Could you check a few things on this model? Use its own coordinates, in mm. A direction names the side the tool comes from. Coordinates: 2 decimals unless noted, no trailing zeros. Order: outer loops, then holes, each group sorted by start corner. A loop starts at its lowest first (then second) coordinate and runs counter-clockwise, first axis right, second up. Notation, with made-up numbers: (34, 22.25) -> (63, 22.25) arc R14 cw to (63, 47.25) -> close; hole circle Ø1 at (-22, 2.25). An arc over 180 degrees is marked (long way). Return JSON: item names as keys, results as strings. Group by question number.
from build123d import *

# Parameters (mm, degrees)
F0_W     = 100
F0_H     = 70
F1_DEPTH = 30
F2_W     = 70
F2_H     = 60
F3_DEPTH = 13.9
F4_W     = 51.206012
F4_H     = 33.682036
F5_DEPTH = 3.8


with BuildPart() as f1:
    # F0 (on Front) → F1 (new body)
    with BuildSketch(Plane.XZ):
        Rectangle(F0_W, F0_H)
    extrude(amount=F1_DEPTH)

    # F2 (on face) → F3 (cut)
    with BuildSketch(Plane.XZ.offset(30)):
        Rectangle(F2_W, F2_H)
    extrude(amount=-F3_DEPTH, mode=Mode.SUBTRACT)

    # F4 (on face) → F5 (cut)
    with BuildSketch(Plane.XZ.offset(16.1)):
        Rectangle(F4_W, F4_H)
    extrude(amount=-F5_DEPTH, mode=Mode.SUBTRACT)


solid = f1.part
Q1. I want a section at B-B on y = -21. Please give me the cut outline in (x, z).
Q2. I want a section at D-D on z = 14.5. Please give me the cut outline in (x, y).
Q3. On a 3-axis mill with a long thin cutter (end or side, diameter ignored), from which of +Z, -Z, +X, -X, +Y, -Y can I reach the whole of each face in a straight line? I mean faces 4 (the flat face through (-1, -30, -31)), 5 (the flat face through (0, -16.1, 20)). Say none if no direction works.
Q4. I want a section at A-A on z = -18. Please give me the cut outline in (x, y).
Q5. I'm going to push flat-ended pins straight in: pin 1 Ø2 at (x, z) = (-12, 20) entering from -Y; pin 2 Ø12 at (x, z) = (-7, 1.5) entering from -Y. Where does each tip first touch, or does it pass through?
Q6. I want a section at C-C on x = 20.5. Please give me the cut outline in (y, z), and give its area (3 significant figures).
Q7. I need wall thicknesses on line 1 along X through (y, z) = (-19.5, -4.5); line 2 along Z through (x, y) = (-21, -12.5); line 3 along Z through (x, y) = (5, -21.75). Which ranges of each line are inside material? Lowest first, please. Write a range as from..to.
Q8. We'd pull the mould along X, two halves only. Please class faces 1 (the flat face through (0, -14, -16.841)), 2 (the flat face through (50, -15, 0)), 3 (the flat face through (-1, 0, 0)): pulls with the +X half, pulls with the -X half, needs draft (parallel to the pull), parting line crosses it, or undercut.
Response values:
{
 "1": {"outline": "(-50, -35) -> (50, -35) -> (50, 35) -> (-50, 35) -> close; hole (-35, -30) -> (35, -30) -> (35, 30) -> (-35, 30) -> close"},
 "2": {"outline": "(-50, -30) -> (-35, -30) -> (-35, -16.1) -> (-25.6, -16.1) -> (-25.6, -12.3) -> (25.6, -12.3) -> (25.6, -16.1) -> (35, -16.1) -> (35, -30) -> (50, -30) -> (50, 0) -> (-50, 0) -> close"},
 "3": {"face 4": "+Z, -Z, +X, -X, -Y", "face 5": "-Y"},
 "4": {"outline": "(-50, -30) -> (-35, -30) -> (-35, -16.1) -> (35, -16.1) -> (35, -30) -> (50, -30) -> (50, 0) -> (-50, 0) -> close"},
 "5": {"pin 1": "stops at y = -16.1", "pin 2": "stops at y = -12.3"},
 "6": {"outline": "(-30, -35) -> (0, -35) -> (0, 35) -> (-30, 35) -> (-30, 30) -> (-16.1, 30) -> (-16.1, 16.84) -> (-12.3, 16.84) -> (-12.3, -16.84) -> (-16.1, -16.84) -> (-16.1, -30) -> (-30, -30) -> close", "area": "1,140 mm²"},
 "7": {"line 1": "x = -50..-35, 35..50", "line 2": "z = -35..-16.84, 16.84..35", "line 3": "z = -35..-30, 30..35"},
 "8": {"face 1": "undercut", "face 2": "pulls with the +X half", "face 3": "needs draft"}
}
